Verification items for the finished model (mm, model axes). A direction names the side the tool comes from. Round coordinates to 2 decimals unless told otherwise and drop trailing zeros. Order: outer loops, then holes, each group sorted by start corner. A loop starts at its lowest first (then second) coordinate and runs counter-clockwise, first axis right, second up. Notation, with made-up numbers: (36, -22) -> (72, -22) arc R13 cw to (72, -8) -> close; hole circle Ø10 at (24, -34.5). An arc over 180 degrees is marked (long way). Return JSON: item names as keys, results as strings. Group by question number.
Item 1: Sectioned sample at D-D on x = 11. Record the cut outline in (y, z), plus the area to 3 significant figures.
Item 2: Access from +Z, -Z, +X, -X, +Y, -Y to the whole of each face (thin tool, end or side, straight path). Record for faces 1 (the flat face through (0, -55, 17)), 2 (the flat face through (-20, 53, 11.918)), 3 (the flat face through (0, -52, 11.918)), 4 (the flat face through (-15, 52, 18)).
Item 3: Depth check by flat-ended pin: pin 1 Ø4 at (x, y) = (-19.5, 53.5) entering from -Z; pin 2 Ø6 at (x, y) = (15, -31) entering from +Z; pin 3 Ø20 at (x, z) = (3, 13) entering from +Y. Enter the tip coordinate at first touch or a pass-through.
Item 4: Scan lines: probe 1 along Y at (x, z) = (16, 2); probe 2 along Y at (x, z) = (-0.5, 12.5); probe 3 along Z at (x, y) = (-17.5, 27). Record each from-to range of solid material in increasing order. Write a range as from..to.
Item 5: Sectioned sample at C-C on y = -42.5. Record the cut outline in (x, z), plus the area to 3 significant figures.
Item 6: Sectioned sample at B-B on x = -17. Record the cut outline in (y, z).
Item 7: Sectioned sample at A-A on z = 19.5. Record the cut outline in (x, y), plus the area to 3 significant figures.
```python
from build123d import *

# Parameters (mm, degrees)
SKETCH1_W           = 50
SKETCH1_H           = 100
BOSS_EXTRUDE1_DEPTH = 20
BOSS_EXTRUDE2_DEPTH = 50
SKETCH3_W           = 30
SKETCH3_H           = 5
CUT_EXTRUDE1_DEPTH  = 30


with BuildPart() as part:
    # Sketch1 → Boss-Extrude1 (new body)
    with BuildSketch(Plane.XY):
        Rectangle(SKETCH1_W, SKETCH1_H)
    extrude(amount=BOSS_EXTRUDE1_DEPTH)

    # Sketch2 → Boss-Extrude2 (add, through all)
    with BuildSketch(Plane(origin=(25, 0, 0), x_dir=(0, 0, -1), z_dir=(1, 0, 0))):
        with BuildLine():
            Line((-11.918313109, 55), (-11.918313109, -55))
            Line((-11.918313109, -55), (-21.936720316, -55))
            ThreePointArc((-21.936720316, -55), (-37.569706847, 0), (-21.936720316, 55))
            Line((-21.936720316, 55), (-11.918313109, 55))
        make_face()
    extrude(amount=-BOSS_EXTRUDE2_DEPTH)

    # Sketch3 → Cut-Extrude1 (cut)
    with BuildSketch(Plane(origin=(0, 0, 0), x_dir=(-1, 0, 0), z_dir=(0, 0, -1))):
        with Locations((0, 52.5)):
            Rectangle(SKETCH3_W, SKETCH3_H)
    extrude(amount=-CUT_EXTRUDE1_DEPTH, mode=Mode.SUBTRACT)


solid = part.part
```
Recorded:
{
 "1": {"outline": "(-55, 11.92) -> (-50, 11.92) -> (-50, 0) -> (50, 0) -> (50, 24.84) arc R104.57 ccw to (-55, 21.94) -> close", "area": "3,400 mm²"},
 "2": {"face 1": "+Z, -Z, +X, -X, -Y", "face 2": "-Z, +X, -X, +Y", "face 3": "-Z, +X, -X, -Y", "face 4": "+Z, -Z, +Y"},
 "3": {"pin 1": "z = 11.92", "pin 2": "z = 33.75", "pin 3": "y = 50"},
 "4": {"probe 1": "-50..50", "probe 2": "-55..50", "probe 3": "0..34.02"},
 "5": {"outline": "(-25, 0) -> (25, 0) -> (25, 28.54) -> (-25, 28.54) -> close", "area": "1,430 mm²"},
 "6": {"outline": "(-55, 11.92) -> (-50, 11.92) -> (-50, 0) -> (50, 0) -> (50, 11.92) -> (55, 11.92) -> (55, 21.94) arc R104.57 ccw to (-55, 21.94) -> close"},
 "7": {"outline": "(-25, -55) -> (25, -55) -> (25, 55) -> (15, 55) -> (15, 50) -> (-15, 50) -> (-15, 55) -> (-25, 55) -> close", "area": "5,350 mm²"}
}
